Geometry check sheet. Reference: the model listing, model coordinates, mm. Face numbers are marked on the shaded views. A direction names the side the tool comes from. Coordinates: 2 decimals unless noted, no trailing zeros. Write each loop counter-clockwise with the first axis right and the second up, starting at its lowest first coordinate (ties: lowest second). Pieces come first, ordered by that corner, then holes. Notation, with made-up numbers: (49.5, -11) -> (99.5, -11) arc R20 ccw to (99.5, 27) -> close; hole circle Ø5 at (-28.5, 24). An arc over 180 degrees is marked (long way). Answer as CSV lines item,"result".
```python
from build123d import *

# Parameters (mm, degrees)
BOX_W        = 7.5
BOX_H        = 13.5
BOX_DEPTH    = 10
FILLET_R     = 0.3
SKETCH_W     = 4.5
SKETCH_H     = 10.5
POCKET_DEPTH = 10


with BuildPart() as part:
    # Box → Box (new body)
    with BuildSketch(Plane.XY):
        with Locations((3.75, 6.75)):
            Rectangle(BOX_W, BOX_H)
    extrude(amount=BOX_DEPTH)

    # Fillet
    fillet_edges = [part.edges().sort_by_distance(p)[0] for p in [
        (0, 0, 5),
        (0, 6.75, 10),
        (0, 13.5, 5),
        (0, 6.75, 0),
        (7.5, 0, 5),
        (7.5, 6.75, 10),
        (7.5, 13.5, 5),
        (7.5, 6.75, 0),
        (3.75, 0, 0),
        (3.75, 0, 10),
        (3.75, 13.5, 0),
        (3.75, 13.5, 10),
    ]]
    fillet(fillet_edges, radius=FILLET_R)

    # Sketch (on Face6 of Box) → Pocket (cut)
    with BuildSketch(Plane.XY.offset(10)):
        with Locations((3.733011, 6.744313)):
            Rectangle(SKETCH_W, SKETCH_H)
    extrude(amount=-POCKET_DEPTH, mode=Mode.SUBTRACT)


solid = part.part
```
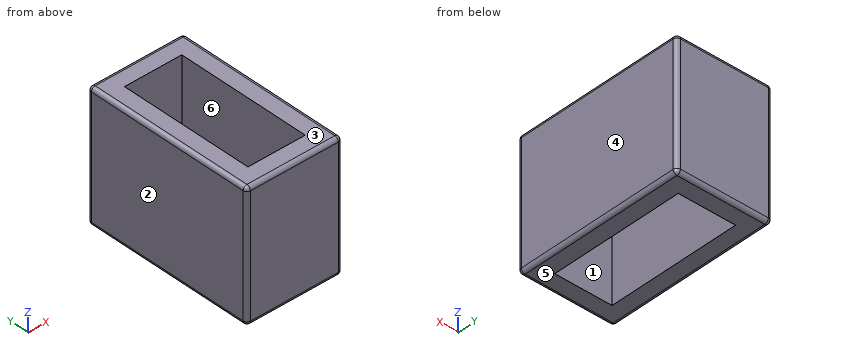
Item 1: Cross-section at C-C, the plane z = 7. Record the cut outline in (x, y), plus the area to 3 significant figures.
Responses:
outline,"(0, 0.3) arc R0.3 ccw to (0.3, 0) -> (7.2, 0) arc R0.3 ccw to (7.5, 0.3) -> (7.5, 13.2) arc R0.3 ccw to (7.2, 13.5) -> (0.3, 13.5) arc R0.3 ccw to (0, 13.2) -> close; hole (1.48, 1.49) -> (5.98, 1.49) -> (5.98, 11.99) -> (1.48, 11.99) -> close"
area,"53.9 mm2"
Item 2: Cross-section at A-A, the plane y = 5. Record the cut outline in (x, z).
Responses:
outline,"(0, 0.3) arc R0.3 ccw to (0.3, 0) -> (1.48, 0) -> (1.48, 10) -> (0.3, 10) arc R0.3 ccw to (0, 9.7) -> close; (5.98, 0) -> (7.2, 0) arc R0.3 ccw to (7.5, 0.3) -> (7.5, 9.7) arc R0.3 ccw to (7.2, 10) -> (5.98, 10) -> close"
Item 3: Set-up check for the marked faces 5 and 6: record each of +Z, -Z, +X, -X, +Y, -Y from which the full face is reachable in a straight line by a thin tool's end or side.
Responses:
face 5,"-Z, +X, -X, +Y, -Y"
face 6,"+Z, -Z"
Item 4: Cross-section at B-B, the plane x = 5.5. Record the cut outline in (y, z), plus the area to 3 significant figures.
Responses:
outline,"(0, 0.3) arc R0.3 ccw to (0.3, 0) -> (1.49, 0) -> (1.49, 10) -> (0.3, 10) arc R0.3 ccw to (0, 9.7) -> close; (11.99, 0) -> (13.2, 0) arc R0.3 ccw to (13.5, 0.3) -> (13.5, 9.7) arc R0.3 ccw to (13.2, 10) -> (11.99, 10) -> close"
area,"29.9 mm2"
Item 5: Release check for a two-part mould opening along X. For the marked faces 1, 2, 3 and 4 record: +X half, -X half, draft (parallel to the pull), parting line (faces both ways), or undercut.
Responses:
face 1,"undercut"
face 2,"-X half"
face 3,"draft"
face 4,"+X half"
Item 6: Thickness scan on probe 1 along Y at (x, z) = (4.5, 9); probe 2 along X at (y, z) = (7, 4.5). Record the ranges inside material, lowest first.
Responses:
probe 1,"y = 0 to 1.49, 11.99 to 13.5"
probe 2,"x = 0 to 1.48, 5.98 to 7.5"
